For this review, take the finished solid that the model builds, in its own axes (mm). Give positions to 0.01 mm unless a question says otherwise; leave off trailing zeros. Write each loop counter-clockwise with the first axis right and the second up, starting at its lowest first coordinate (ties: lowest second). Pieces come first, ordered by that corner, then holes. Notation, with made-up numbers: (82.5, 45.5) -> (101.5, 45.5) arc R13 ccw to (101.5, 70.5) -> close; hole circle Ø3 at (-10, 59). An arc over 180 degrees is marked (long way). Answer as CSV lines item,"result".
```python
from build123d import *

# Parameters (mm, degrees)
SKETCH3_W = 0.254
SKETCH3_H = 0.508


with BuildPart() as part:
    # Sketch1 → Revolve1 (revolve)
    with BuildSketch(Plane.XY):
        Polygon((0, 0), (0, 1.5875), (1291.463, 1.5875), (1291.463, 4.03225), (1303.3248, 4.03225), (1303.3248, 0), align=None)
    revolve(axis=Axis((1303.3248, 0, 0), (-1, 0, 0)))

    # Sketch2 → Revolve2 (revolve)
    with BuildSketch(Plane.XY):
        Polygon((-9.652, 0), (-9.652, 1.20904), (-9.27354, 1.5875), (0, 1.5875), (0, 0), align=None)
    revolve(axis=Axis((0, 0, 0), (-1, 0, 0)))

    # Sketch3 → Cut-Revolve1 (revolve, cut)
    with BuildSketch(Plane.XY):
        with Locations((-0.127, 1.5875)):
            Rectangle(SKETCH3_W, SKETCH3_H)
    revolve(axis=Axis((0, 0, 0), (-1, 0, 0)), mode=Mode.SUBTRACT)


solid = part.part
```
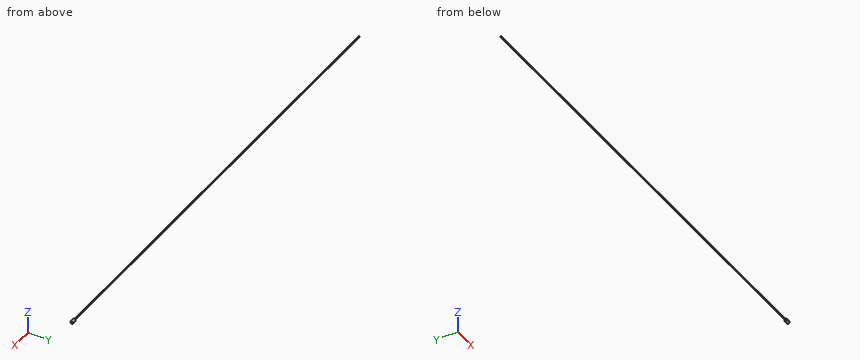
Q1. Clearance check with a flat-ended pin moving along its axis: pin 1 (4 mm diameter, centred on x = 1131.5, y = 2.5, fed in from -Z). State where the tip first meets the part, or that it passes through.
Answer block:
pin 1,"stops at z = -1.51"
Q2. To check wall thickness, follow probe 1 along Z at (x, y) = (964, 0); probe 2 along X at (y, z) = (-1.5, -3.25); probe 3 along Z at (x, y) = (624.5, -1). State the ranges of each line that lie inside material, in increasing order. Write a range as [from, to].
Answer block:
probe 1,"z = [-1.59, 1.59]"
probe 2,"x = [1291.46, 1303.32]"
probe 3,"z = [-1.23, 1.23]"
Q3. Add section A-A (x = 786). Write out the cut boundary in (y, z) (1 decimal).
Answer block:
outline,"circle Ø3.2 at (0, 0)"
